Verification items for the finished model (mm, model axes). Coordinates: 2 decimals unless noted, no trailing zeros. Write each loop counter-clockwise with the first axis right and the second up, starting at its lowest first coordinate (ties: lowest second). Pieces come first, ordered by that corner, then holes. Notation, with made-up numbers: (62.25, 43.5) -> (104.25, 43.5) arc R17 ccw to (104.25, 76.5) -> close; hole circle Ø11 at (23.25, 48). An arc over 180 degrees is marked (long way). Answer in a Markdown table with one row per item.
Autodesk Inventor part; units mm, degrees
ref_plane "YZ Plane" through (0, 0, 0) normal (1, 0, 0) x (0, 1, 0)
ref_plane "XZ Plane" through (0, 0, 0) normal (0, 1, 0) x (-1, 0, 0)
ref_plane "XY Plane" through (0, 0, 0) normal (0, 0, 1) x (1, 0, 0)
sketch "Sketch1" plane through (0, 0, 0) normal (0, 0, 1) x (1, 0, 0)
  line L0 (-12.7, 12.7) -> (-12.7, -12.7)
  line L1 (-12.7, -12.7) -> (12.7, -12.7)
  line L2 (12.7, -12.7) -> (12.7, 12.7)
  line L3 (12.7, 12.7) -> (-12.7, 12.7)
  line L4 (-9.525, 9.525) -> (-9.525, -9.525)
  line L5 (-9.525, -9.525) -> (9.525, -9.525)
  line L6 (9.525, -9.525) -> (9.525, 9.525)
  line L7 (9.525, 9.525) -> (-9.525, 9.525)
  point P0 (0, 0)
  dimension "d0" = 25.4
  dimension "d1" = 25.4
  dimension "d2" = 12.7
  dimension "d3" = 12.7
  dimension "d4" = 3.175
extrude "Extrusion1" add sketch "Sketch1" along normal blind 698.5
properties part number "27 in sq frame"
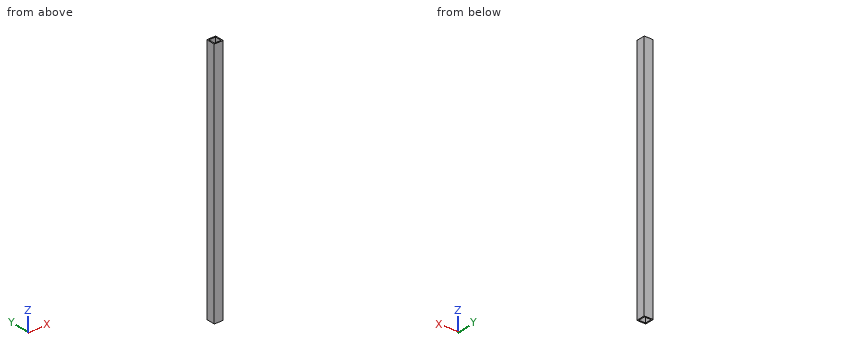
1. Sectioned sample at C-C, the plane z = 395.5. Record the cut outline in (x, y) (3 decimals).
Findings below:
| item | result |
|---|---|
| outline | (-12.7, -12.7) -> (12.7, -12.7) -> (12.7, 12.7) -> (-12.7, 12.7) -> close; hole (-9.525, -9.525) -> (9.525, -9.525) -> (9.525, 9.525) -> (-9.525, 9.525) -> close |
2. Material ranges on probe 1 along Y at (x, z) = (2.5, 478.5) (3 decimals), recorded low to high. Write a range as from..to.
Findings below:
| item | result |
|---|---|
| probe 1 | y = -12.7..-9.525, 9.525..12.7 |
3. Go/stop test with a flat-tipped pin: pin 1 (2 mm diameter, centred on x = 7.5, y = -5, fed in from +Z). Record where the tip stops, or that it passes through.
Findings below:
| item | result |
|---|---|
| pin 1 | passes through |
4. Sectioned sample at A-A, the plane x = -2. Record the cut outline in (y, z) (3 decimals).
Findings below:
| item | result |
|---|---|
| outline | (-12.7, 0) -> (-9.525, 0) -> (-9.525, 698.5) -> (-12.7, 698.5) -> close; (9.525, 0) -> (12.7, 0) -> (12.7, 698.5) -> (9.525, 698.5) -> close |
